from build123d import *

# Parameters (mm, degrees)
PAD_DEPTH       = 8
PAD001_DEPTH    = 8
POCKET_DEPTH    = 2
POCKET001_DEPTH = 2


with BuildPart() as part:
    # Sketch → Pad (new body)
    with BuildSketch(Plane.XY):
        with BuildLine():
            ThreePointArc((0, 30), (5, 35), (0, 40))
            Line((0, 40), (0, 45))
            ThreePointArc((10, 35.000023), (7.07106, 42.071076), (0, 45))
            Line((10, 35.000023), (10, 0))
            Line((10, 0), (0, 0))
            Line((0, 0), (0, 30))
        make_face()
    pad = extrude(amount=PAD_DEPTH)

    # Sketch001 → Pad001 (join)
    with BuildSketch(Plane.XZ):
        with BuildLine():
            Line((0, 0), (10, 0))
            Line((10, 0), (10, 27))
            ThreePointArc((10, 27), (7.071068, 34.071068), (0, 37))
            Line((0, 31.2), (0, 37))
            ThreePointArc((0, 22.8), (4.2, 27), (0, 31.2))
            Line((0, 22.8), (0, 0))
        make_face()
    pad001 = extrude(amount=-PAD001_DEPTH)

    # Sketch002 → Pocket (cut)
    with BuildSketch(Plane(origin=(0, 35, 8), x_dir=(1, 0, 0), z_dir=(0, 0, 1))):
        Polygon((8.082904, 0), (4.041452, 7), (-4.041452, 7), (-8.082904, 0), (-4.041452, -7), (4.041452, -7), align=None)
    pocket = extrude(amount=-POCKET_DEPTH, mode=Mode.SUBTRACT)

    # Sketch003 → Pocket001 (cut)
    with BuildSketch(Plane(origin=(0, 0, 27), x_dir=(1, 0, 0), z_dir=(0, -1, 0))):
        Polygon((3.752777, 6.5), (-3.752777, 6.5), (-7.505553, 0), (-3.752777, -6.5), (3.752777, -6.5), (7.505553, 0), align=None)
    pocket001 = extrude(amount=-POCKET001_DEPTH, mode=Mode.SUBTRACT)

    # Mirrored: Pad, Pad001, Pocket, Pocket001 across Sketch V_Axis
    add(pad.mirror(Plane(origin=(0, 0, 0), x_dir=(0, 0, 1), z_dir=(1, 0, 0))))
    add(pad001.mirror(Plane(origin=(0, 0, 0), x_dir=(0, 0, 1), z_dir=(1, 0, 0))))
    add(pocket.mirror(Plane(origin=(0, 0, 0), x_dir=(0, 0, 1), z_dir=(1, 0, 0))), mode=Mode.SUBTRACT)
    add(pocket001.mirror(Plane(origin=(0, 0, 0), x_dir=(0, 0, 1), z_dir=(1, 0, 0))), mode=Mode.SUBTRACT)


solid = part.part
Here's how the part is built. I have some questions about the finished solid (model axes, mm). A direction names the side the tool comes from. Round coordinates to 2 decimals unless told otherwise and drop trailing zeros. Loops run counter-clockwise (first coordinate to the right, second up) from the corner with the lowest first, then second, coordinate; pieces in that order, holes last.
1. We'd pull the mould along Z, two halves only. Please class faces 6 (the face through (-0.185, 4.958, 31.196)), 7 (the face through (-10, 14, 7)), 8 (the face through (0, 23, 8)): +Z half, -Z half, draft (parallel to the pull), parting line (faces both ways), or undercut.
Answer list:
face 6: undercut
face 7: draft
face 8: +Z half
2. Which directions (+Z, -Z, +X, -X, +Y, -Y) give clear straight access to the entire face, cutting with the end or side of a thin tool? Please do faces 1 (the face through (0, 0, 14)), 2 (the face through (0, 42, 7)), 3 (the face through (-5.6, 1, 23.7)), 4 (the face through (0, 8, 19)), 5 (the face through (10, 14, 7)).
Answer list:
face 1: +Z, -Z, +X, -X, -Y
face 2: +Z
face 3: -Y
face 4: +Z, +X, -X, +Y
face 5: +Z, -Z, +X, +Y, -Y
3. If we section it at A-A on x = -2: Write out the boundary of the cut face in (y, z).
Answer list:
outline: (0, 0) - (30.42, 0) - (30.42, 6) - (28, 6) - (28, 8) - (8, 8) - (8, 23.31) - (2, 23.31) - (2, 20.5) - (0, 20.5) - close; (0, 33.5) - (2, 33.5) - (2, 30.69) - (8, 30.69) - (8, 36.8) - (0, 36.8) - close; (39.58, 0) - (44.8, 0) - (44.8, 8) - (42, 8) - (42, 6) - (39.58, 6) - close
4. For P1, Ø1, axis at x = -1.5, z = 6.5, coming from the +Y side; P2, Ø6, axis at y = 37, z = 7, coming from the -X side; P3, Ø10, axis at x = -3, y = 33, coming from the +Z side; P4, Ø10, axis at x = 4.5, z = 20, coming from the +Y side, each with a flat end and sliding along its axis, tell me the tip position at first contact or that it passes through.
Answer list:
P1: stops at y = 44.95
P2: stops at x = -10
P3: stops at z = 8
P4: stops at y = 8
5. If I drill on line 1 along X through (y, z) = (35, 4); line 2 along Z through (x, y) = (3.25, 28.5); line 3 along Y through (x, z) = (3, 21.5), over which ranges is the centre line in solid material (lowest first)?
Answer list:
line 1: x = -10 to -5, 5 to 10
line 2: z = 0 to 6
line 3: y = 2 to 8
6. If we section it at C-C on y = 23.5: Write out the boundary of the cut face in (x, z).
Answer list:
outline: (-10, 0) - (10, 0) - (10, 8) - (-10, 8) - close
7. If we section it at B-B on y = 38: Write out the boundary of the cut face in (x, z).
Answer list:
outline: (-9.54, 0) - (-4, 0) - (-4, 6) - (-6.35, 6) - (-6.35, 8) - (-9.54, 8) - close; (4, 0) - (9.54, 0) - (9.54, 8) - (6.35, 8) - (6.35, 6) - (4, 6) - close
